```python
from build123d import *

# Parameters (mm, degrees)
BOSS_EXTRUDE1_DEPTH = 5
SKETCH3_W           = 8
SKETCH3_H           = 4
BOSS_EXTRUDE2_DEPTH = 3
FILLET1_START       = -3.841593316
FILLET1_DEPTH       = 8
CUT_EXTRUDE1_START  = -10
CUT_EXTRUDE1_DEPTH  = 10
FILLET2_R           = 3
SKETCH6_R           = 1.5
CUT_EXTRUDE2_DEPTH  = 5


with BuildPart() as part:
    # Sketch1 → Boss-Extrude1 (new body)
    with BuildSketch(Plane(origin=(0, 0, 0), x_dir=(1, 0, 0), z_dir=(0, 1, 0))):
        with BuildLine():
            Line((-30, 0), (30, 0))
            ThreePointArc((30, 0), (0, 30), (-30, 0))
        make_face()
    extrude(amount=BOSS_EXTRUDE1_DEPTH)

    # Sketch3 → Boss-Extrude2 (add)
    with BuildSketch(Plane(origin=(0, 5, 0), x_dir=(1, 0, 0), z_dir=(0, 1, 0))):
        with Locations((0.158406684, 24.731666579)):
            Rectangle(SKETCH3_W, SKETCH3_H)
    extrude(amount=BOSS_EXTRUDE2_DEPTH)

    # Fillet1: read off the stored shape, not the designer's step
    # Fillet1 outline → Fillet1 (cut)
    with BuildSketch(Plane.YZ.offset(FILLET1_START)):
        with BuildLine():
            Line((8, -22.731666579), (5, -22.731666579))
            add(Edge.make_bspline(
                [(5, -22.731666579), (8, -23.506263249), (8, -26.604649926)],
                knots=[0, 0, 0, 1, 1, 1], degree=2, weights=[1, 0.057495957, 1]))
            Line((8, -26.604649926), (8, -22.731666579))
        make_face()
    extrude(amount=FILLET1_DEPTH, mode=Mode.SUBTRACT)

    # Sketch5 → Cut-Extrude1 (cut)
    with BuildSketch(Plane(origin=(0, 5, 0), x_dir=(1, 0, 0), z_dir=(0, 1, 0)).offset(CUT_EXTRUDE1_START)):
        with BuildLine():
            Line((-21.393876913, 0), (-21.393876913, 6))
            Line((-21.393876913, 6), (-29.393876913, 6))
            ThreePointArc((-29.393876913, 6), (-29.84808459, 3.01526886), (-30, 0))
            Line((-30, 0), (-21.393876913, 0))
        make_face()
        with BuildLine():
            Line((21.393876913, 6), (29.393876913, 6))
            ThreePointArc((29.393876913, 6), (29.84808459, 3.01526886), (30, 0))
            Line((30, 0), (21.393876913, 0))
            Line((21.393876913, 0), (21.393876913, 6))
        make_face()
    extrude(amount=CUT_EXTRUDE1_DEPTH, mode=Mode.SUBTRACT)

    # Fillet2
    fillet2_edges = [part.edges().sort_by_distance(p)[0] for p in [
        (0, 5, 0),
    ]]
    fillet(fillet2_edges, radius=FILLET2_R)

    # Sketch6 → Cut-Extrude2 (cut)
    with BuildSketch(Plane(origin=(21.393876913, 0, 0), x_dir=(0, 0, -1), z_dir=(1, 0, 0))):
        with Locations((3, 2.25)):
            Circle(SKETCH6_R)
    extrude(amount=-CUT_EXTRUDE2_DEPTH, mode=Mode.SUBTRACT)


solid = part.part
```
Work out the finished part from the listing and answer in its coordinate system (mm). A direction names the side the tool comes from. Give positions to 0.01 mm unless a question says otherwise; leave off trailing zeros. Loops run counter-clockwise (first coordinate to the right, second up) from the corner with the lowest first, then second, coordinate; pieces in that order, holes last. Notation, with made-up numbers: M 39.5,-15 L 93.5,-15 A29 ccw 93.5,13 Z; hole C 79.25,48.25 d7. An arc over 180 degrees is marked long. One line per item, written item: value. Start each with the question number.
1. Find section C-C (x = 25.5). Give the vertices of the cut face in (y, z), and give its area (3 significant figures).
2. Find the intervals of material crossed by probe 1 along Y at (x, z) = (6.5, -7); probe 2 along X at (y, z) = (6, -25.75); probe 3 along X at (y, z) = (3.25, -3.5), in increasing order.
3. Which of the six approach directions +Z, -Z, +X, -X, +Y, -Y give full straight-line access (tool end or side, diameter ignored) to faces 5 (the face through (-25, 2, -6)), 6 (the face through (18.93, 0.92, -3.69)), 7 (the face through (4.158, 6, -25))?
4. Find section A-A (x = -16). Give the vertices of the cut face in (y, z), and give its area (3 significant figures).
5. Determine the mould class of faces 1 (the face through (0, 6, -26.732)), 2 (the face through (16.394, 2, -3)), 3 (the face through (25, 2, -6)), 4 (the face through (-21.394, 2, -3)) for opening direction Z: released by +Z, released by -Z, zero draft, split by the parting line, or undercut.
6. Each of these flat-tipped pins is pushed along its axis until it touches: P1, Ø0.9, axis at y = 2.5, z = -3, coming from the +X side; P2, Ø8, axis at x = 4, z = -19, coming from the +Y side; P3, Ø2, axis at y = 3, z = -10.5, coming from the -X side. Where does it stop, or does it pass through?
7. Find section B-B (z = -13.75). Give the vertices of the cut face in (x, y).
8. Find section D-D (x = -4.5). Give the vertices of the cut face in (y, z).
Reported:
1. outline: M 0,-15.8 L 5,-15.8 L 5,-6 L 0,-6 Z
1. area: 49.0 mm²
2. probe 1: y = 0 to 5
2. probe 2: x = -3.84 to 4.16
2. probe 3: x = -21.39 to 16.39
3. face 5: +Z, -X, +Y, -Y
3. face 6: +X
3. face 7: +Z, -Z, +X, +Y
4. outline: M 0,-25.38 L 5,-25.38 L 5,-3 A3 ccw 2,0 L 0,0 Z
4. area: 125 mm²
5. face 1: released by -Z
5. face 2: undercut
5. face 3: released by +Z
5. face 4: zero draft
6. P1: stops at x = 16.39
6. P2: stops at y = 5.27
6. P3: stops at x = -28.46
7. outline: M -26.66,0 L 26.66,0 L 26.66,5 L -26.66,5 Z
8. outline: M 0,-29.66 L 5,-29.66 L 5,-3 A3 ccw 2,0 L 0,0 Z
